Can you work these out from the model? Positions are in its coordinate system, mm. A direction names the side the tool comes from. Round coordinates to 2 decimals unless told otherwise and drop trailing zeros. Order: outer loops, then holes, each group sorted by start corner. A loop starts at its lowest first (then second) coordinate and runs counter-clockwise, first axis right, second up.
Q1. If we section it at D-D (x = 3.75): Please give me the cut outline in (y, z).
Q2. If we section it at B-B (y = -4.75): Please give me the cut outline in (x, z), plus the area to 3 significant figures.
Q3. If we section it at C-C (z = 11): Please give me the cut outline in (x, y), plus the area to 3 significant figures.
Q4. Will this pin go through, and if not, where does the flat tip stop? P1, Ø1.5, axis at x = 0.5, z = 10, coming from the -Y side.
Q5. If I drill on line 1 (Y direction, x = -8.75, z = 7); line 2 (X direction, y = -0.75, z = 34.5); line 3 (X direction, y = 5.25, z = 43.5), over which ranges is the centre line in solid material (lowest first)?
Q6. We'd pull the mould along Y, two halves only. Please class faces 1 (the face through (-8.99, -1, 25)), 2 (the face through (6.34, -4, 25)), 3 (the face through (10, 5.9, 25)): pulls with the +Y half, pulls with the -Y half, needs draft (parallel to the pull), parting line crosses it, or undercut.
Q7. If we section it at A-A (x = 8.5): Please give me the cut outline in (y, z), plus the area to 3 significant figures.
Q8. For faces 4 (the face through (8, -2.83, 25)), 5 (the face through (-6.34, -4, 25)), 6 (the face through (4.111, 4.633, 24.65)), which set-ups out of +Z, -Z, +X, -X, +Y, -Y let a thin tool reach every point of the face, with its end or its side?
from build123d import *

# Parameters (mm, degrees)
F0_W     = 2.65
F0_H     = 3.07
F1_DEPTH = 50


with BuildPart() as f1:
    # F0 (on Top) → F1 (new body)
    with BuildSketch(Plane.XY):
        Polygon((-8.99, 0.489908), (-11.843405, 0.489908), (-11.843405, -5.900092), (-8.99, -5.900092), (-8.99, -2.830092), align=None)
        Polygon((-7.843405, 5.900092), (-11.843405, 5.900092), (-11.843405, 0.489908), (-8.99, 0.489908), (8.99, 0.489908), (11.843405, 0.489908), (11.843405, 5.900092), (7.843405, 5.900092), (5.343405, 3.400092), (2.843405, 5.900092), (-2.843405, 5.900092), (-5.343405, 3.400092), align=None)
        Polygon((11.843405, 0.489908), (8.99, 0.489908), (8.99, -2.830092), (8.99, -5.900092), (11.843405, -5.900092), align=None)
        with Locations((7.665, -4.365092)):
            Rectangle(F0_W, F0_H)
        with Locations((-7.665, -4.365092)):
            Rectangle(F0_W, F0_H)
    extrude(amount=F1_DEPTH)


solid = f1.part
Solution:
1. outline: (0.49, 0) - (4.99, 0) - (4.99, 50) - (0.49, 50) - close
2. outline: (-11.84, 0) - (-6.34, 0) - (-6.34, 50) - (-11.84, 50) - close; (6.34, 0) - (11.84, 0) - (11.84, 50) - (6.34, 50) - close
2. area: 550 mm2
3. outline: (-11.84, -5.9) - (-6.34, -5.9) - (-6.34, -2.83) - (-8.99, -2.83) - (-8.99, 0.49) - (8.99, 0.49) - (8.99, -2.83) - (6.34, -2.83) - (6.34, -5.9) - (11.84, -5.9) - (11.84, 5.9) - (7.84, 5.9) - (5.34, 3.4) - (2.84, 5.9) - (-2.84, 5.9) - (-5.34, 3.4) - (-7.84, 5.9) - (-11.84, 5.9) - close
3. area: 168 mm2
4. P1: stops at y = 0.49
5. line 1: y = -5.9 to -2.83, 0.49 to 5.9
5. line 2: x = -11.84 to -8.99, 8.99 to 11.84
5. line 3: x = -11.84 to -7.19, -3.49 to 3.49, 7.19 to 11.84
6. face 1: undercut
6. face 2: needs draft
6. face 3: pulls with the +Y half
7. outline: (-5.9, 0) - (-2.83, 0) - (-2.83, 50) - (-5.9, 50) - close; (0.49, 0) - (5.9, 0) - (5.9, 50) - (0.49, 50) - close
7. area: 424 mm2
8. face 4: +Z, -Z
8. face 5: +Z, -Z, -Y
8. face 6: +Z, -Z, +Y
